The model under review builds one solid part; all positions refer to its coordinate system, in mm. Face numbers are marked on the shaded views. A direction names the side the tool comes from. Round coordinates to 2 decimals unless told otherwise and drop trailing zeros. Loops run counter-clockwise (first coordinate to the right, second up) from the corner with the lowest first, then second, coordinate; pieces in that order, holes last. Notation, with made-up numbers: M 16,13.5 L 29,13.5 A25 ccw 29,25.5 Z; hole C 18,71.25 d1. An arc over 180 degrees is marked long. Return JSON: item names as keys, results as strings. Group by question number.
Q1. To check wall thickness, follow line 1 along Y through (x, z) = (-4.5, 0); line 2 along Y through (x, z) = (-22, 0.5); line 3 along X through (y, z) = (-80, 2). State the ranges of each line that lie inside material, in increasing order.
Q2. Consider section D-D (x = 23.5). State the section outline as (y, z) points, and give its area (3 significant figures).
Q3. Consider section A-A (x = 0). State the section outline as (y, z) points, and give its area (3 significant figures).
Q4. Clearance check with flat-ended pins moving along their axes: pin 1 Ø5.5 at (y, z) = (-175, 0) entering from -X; pin 2 Ø6 at (x, z) = (11, 20) entering from +Y; pin 3 Ø6.5 at (y, z) = (175, 0) entering from +X. State where each tip first meets the part, or that it passes through.
Q5. Consider section C-C (z = -22). State the section outline as (x, y) points.
Q6. Consider section B-B (y = -19.5). State the section outline as (x, z) points, and give its area (3 significant figures).
Q7. For the marked faces 1, 2 and 3, list the 3-axis set-ups (+Z, -Z, +X, -X, +Y, -Y) from which the entire face can be reached by the end or side of a thin tool; tool diameter is ignored.
Autodesk Inventor part; units mm, degrees
ref_plane "Work Plane1" through (-9, 135, 0) normal (-1, 0, 0) x (0, 1, 0)
ref_plane "YZ Plane" through (0, 0, 0) normal (1, 0, 0) x (0, 1, 0)
ref_plane "XZ Plane" through (0, 0, 0) normal (0, 1, 0) x (-1, 0, 0)
sketch "Sketch1" plane through (0, 0, 0) normal (0, 1, 0) x (-1, 0, 0)
  circle A0 centre (0, 0) radius 30
  dimension "d0" = 60
extrude "Extrusion1" add sketch "Sketch1" along normal mid plane 270
sketch "Sketch2" plane through (0, -135, 0) normal (0, -1, 0) x (1, 0, 0)
  circle A0 centre (0, 0) radius 8.5
  dimension "d3" = 17
extrude "Extrusion2" add sketch "Sketch2" along normal blind 50
sketch "Sketch3" plane through (0, 135, 0) normal (0, 1, 0) x (1, 0, 0)
  circle A0 centre (0, 0) radius 8.5
  circle A1 centre (0, 0) radius 8.5
  dimension "d6" = 17
extrude "Extrusion3" add sketch "Sketch3" along normal blind 50
ref_plane "Work Plane1" through (-9, 135, 0) normal (-1, 0, 0) x (0, 1, 0)
sketch "Sketch4" plane through (-9, 135, 0) normal (-1, 0, 0) x (0, 1, 0)
  circle A0 centre (40, 0) radius 4
  circle A1 centre (-310, 0) radius 4
  point P0 (-135, 0)
hole "Hole1" at (-9, 175, 0) at (-9, -175, 0) direction (1, 0, 0) diameter 4.917 end through all
properties part number "HCMUTE-CDT23-TRUC_CANG" material "Stainless Steel"
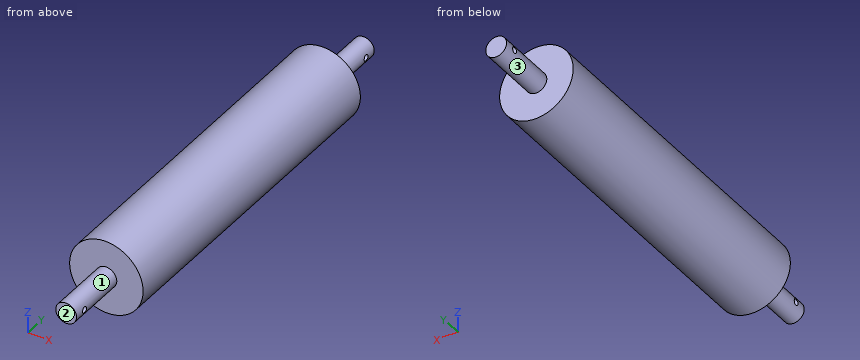
Values:
{
 "1": {"line 1": "y = -185 to -177.46, -172.54 to 172.54, 177.46 to 185", "line 2": "y = -135 to 135", "line 3": "x = -29.93 to 29.93"},
 "2": {"outline": "M -135,-18.65 L 135,-18.65 L 135,18.65 L -135,18.65 Z", "area": "10,100 mm2"},
 "3": {"outline": "M -185,-8.5 L -135,-8.5 L -135,-30 L 135,-30 L 135,-8.5 L 185,-8.5 L 185,8.5 L 135,8.5 L 135,30 L -135,30 L -135,8.5 L -185,8.5 Z; hole C -175,0 d4.92; hole C 175,0 d4.92", "area": "17,900 mm2"},
 "4": {"pin 1": "stops at x = -8.5", "pin 2": "stops at y = 135", "pin 3": "stops at x = 8.5"},
 "5": {"outline": "M -20.4,-135 L 20.4,-135 L 20.4,135 L -20.4,135 Z"},
 "6": {"outline": "C 0,0 d60", "area": "2,830 mm2"},
 "7": {"face 1": "-Y", "face 2": "+Z, -Z, +X, -X, -Y", "face 3": "+Y"}
}
